Source: three-view drawing plus pictorial views. Frame: mm from the lowest corner of the part. A direction names the side the tool comes from. Give positions to 0.01 mm unless a question says otherwise; leave off trailing zeros. Write each loop counter-clockwise with the first axis right and the second up, starting at its lowest first coordinate (ties: lowest second). Pieces come first, ordered by that corner, then holes. Notation, with made-up numbers: M 40,16 L 72,16 A23 cw 72,32 Z; hole C 75.25,42.5 d5. An arc over 180 degrees is marked long. Return JSON: item names as keys, results as strings.
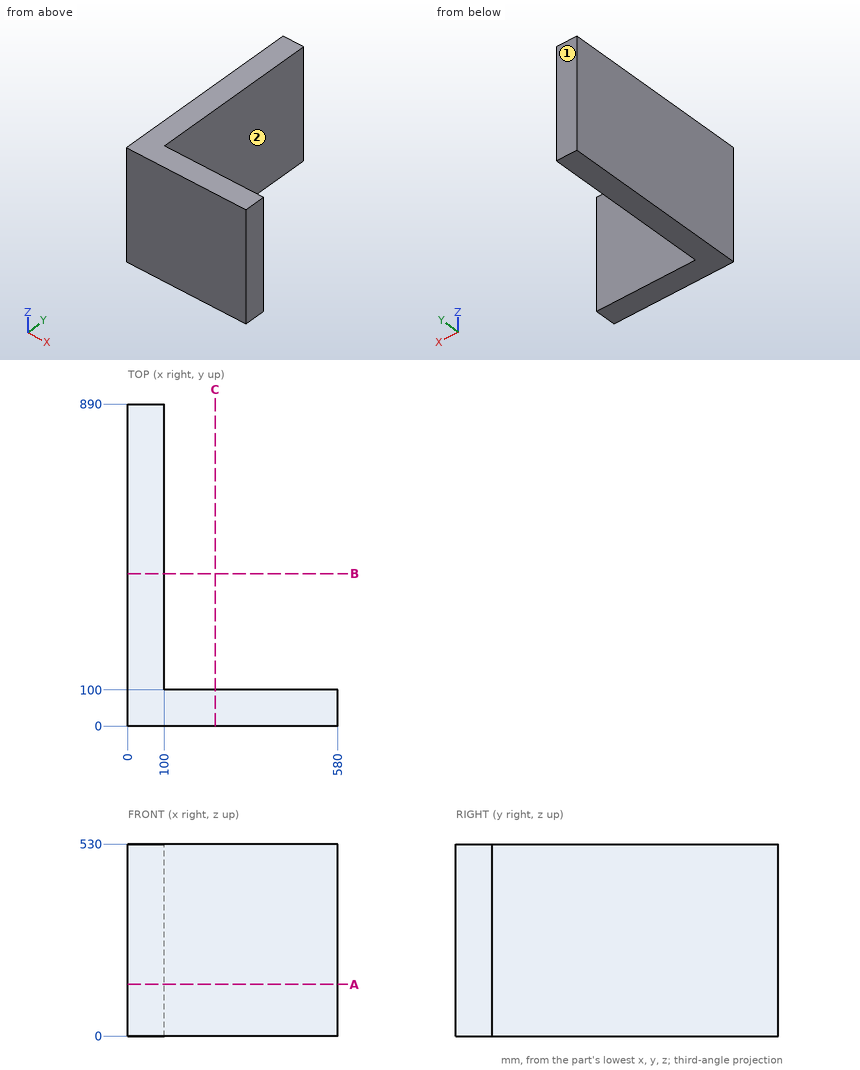
1) Cut plane A-A, the plane z = 142.5. Return the cut outline in (x, y).
Numbers:
{"outline": "M 0,0 L 580,0 L 580,100 L 100,100 L 100,890 L 0,890 Z"}
2) Cut plane B-B, the plane y = 421.5. Return the cut outline in (x, z).
Numbers:
{"outline": "M 0,0 L 100,0 L 100,530 L 0,530 Z"}
3) Contact query for flat-ended pins moving along their axis: pin 1 Ø10 at (y, z) = (299.5, 53.5) entering from +X; pin 2 Ø6 at (x, z) = (331.5, 82.5) entering from +Y. Output: stop coordinate, or through.
Numbers:
{"pin 1": "stops at x = 100", "pin 2": "stops at y = 100"}
4) Set-up query: the marked faces 1 and 2. Return all of +Z, -Z, +X, -X, +Y, -Y with unobstructed straight access to the full face (end or side cutting, diameter ignored); none if empty.
Numbers:
{"face 1": "+Z, -Z, +X, -X, +Y", "face 2": "+Z, -Z, +X, +Y"}
5) Line query: line 1 (X direction, y = 304.5, z = 135.5). Output: solid intervals per line, ascending. Write a range as [from, to].
Numbers:
{"line 1": "x = [0, 100]"}
